from build123d import *

# Parameters (mm, degrees)
BOSS_EXTRUDE1_DEPTH           = 5
SHELL1_T                      = -1
BOSS_EXTRUDE2_DEPTH           = 3.5
CBORE_FOR_M2_SHCS1_AT_2_COUNT = 2
CBORE_FOR_M2_SHCS1_AT_2_PITCH = 23.999204153
FILLET1_R                     = 0.5
SKETCH5_R                     = 5.5
CUT_EXTRUDE1_DEPTH            = 10


with BuildPart() as part:
    # Sketch1 → Boss-Extrude1 (new body)
    with BuildSketch(Plane.XY):
        with BuildLine():
            ThreePointArc((-3.835922715, 7.919955614), (-5.100340344, 7.171229209), (-6.222539674, 6.222539674))
            Line((-6.222539674, 6.222539674), (6.222539674, -6.222539674))
            ThreePointArc((6.222539674, -6.222539674), (7.171229209, -5.100340344), (7.919955614, -3.835922715))
            ThreePointArc((7.919955614, -3.835922715), (8.577167639, -1.967789445), (8.8, 0))
            ThreePointArc((8.8, 0), (4.67353614, 7.456410661), (-3.835922715, 7.919955614))
        make_face()
        with BuildLine():
            Line((6.222539674, -6.222539674), (-6.222539674, 6.222539674))
            ThreePointArc((-6.222539674, 6.222539674), (-7.171229209, 5.100340344), (-7.919955614, 3.835922715))
            ThreePointArc((-7.919955614, 3.835922715), (-6.222539674, -6.222539674), (3.835922715, -7.919955614))
            ThreePointArc((3.835922715, -7.919955614), (5.100340344, -7.171229209), (6.222539674, -6.222539674))
        make_face()
    extrude(amount=BOSS_EXTRUDE1_DEPTH)

    # Shell1
    shell1_openings = [part.faces().sort_by_distance(p)[0] for p in [
        (0, 0, 0),
    ]]
    offset(amount=SHELL1_T, openings=shell1_openings, kind=Kind.INTERSECTION)

    # Sketch1_4 → Boss-Extrude2 (add)
    with BuildSketch(Plane.XY):
        with BuildLine():
            ThreePointArc((-7.919955614, 3.835922715), (-7.171229209, 5.100340344), (-6.222539674, 6.222539674))
            ThreePointArc((-6.222539674, 6.222539674), (-5.100340344, 7.171229209), (-3.835922715, 7.919955614))
            Line((-3.835922715, 7.919955614), (-8.49355603, 12.577588929))
            Line((-8.49355603, 12.577588929), (-12.577588929, 8.49355603))
            Line((-12.577588929, 8.49355603), (-7.919955614, 3.835922715))
        make_face()
        with BuildLine():
            ThreePointArc((7.919955614, -3.835922715), (7.171229209, -5.100340344), (6.222539674, -6.222539674))
            ThreePointArc((6.222539674, -6.222539674), (5.100340344, -7.171229209), (3.835922715, -7.919955614))
            Line((3.835922715, -7.919955614), (8.49355603, -12.577588929))
            Line((8.49355603, -12.577588929), (12.577588929, -8.49355603))
            Line((12.577588929, -8.49355603), (7.919955614, -3.835922715))
        make_face()
    extrude(amount=BOSS_EXTRUDE2_DEPTH)

    # Sketch4 → CBORE for M2 SHCS1 (revolve, cut)
    with BuildSketch(Plane(origin=(-8.485, 8.485, 3.5), x_dir=(0, -1, 0), z_dir=(1, 0, 0))):
        Polygon((0, 0), (0, 3.5), (1.2, 3.5), (1.2, 2), (2.2, 2), (2.2, 0.025), (2.225, 0), align=None)
    cbore_for_m2_shcs1 = revolve(axis=Axis((-8.485, 8.485, 9.85), (0, 0, -1)), mode=Mode.SUBTRACT)

    # CBORE for M2 SHCS1 at 2: CBORE for M2 SHCS1 ×2
    with Locations(*[Vector(0.7071067811865476, -0.7071067811865476, 0) * (i * CBORE_FOR_M2_SHCS1_AT_2_PITCH) for i in range(1, CBORE_FOR_M2_SHCS1_AT_2_COUNT)]):
        add(cbore_for_m2_shcs1, mode=Mode.SUBTRACT)

    # Fillet1
    fillet1_edges = [part.edges().sort_by_distance(p)[0] for p in [
        (6.164739372, -10.248772271, 3.5),
        (8.49355603, -12.577588929, 1.75),
        (12.577588929, -8.49355603, 1.75),
        (10.535572479, -10.535572479, 3.5),
        (10.248772271, -6.164739372, 3.5),
        (-12.577588929, 8.49355603, 1.75),
        (-6.164739372, 10.248772271, 3.5),
        (-8.49355603, 12.577588929, 1.75),
        (-10.248772271, 6.164739372, 3.5),
        (-10.535572479, 10.535572479, 3.5),
        (6.222539674, -6.222539674, 5),
    ]]
    fillet(fillet1_edges, radius=FILLET1_R)

    # Sketch5 → Cut-Extrude1 (cut)
    with BuildSketch(Plane.XY.offset(5)):
        Circle(SKETCH5_R)
    extrude(amount=-CUT_EXTRUDE1_DEPTH, mode=Mode.SUBTRACT)


solid = part.part
For this review, take the finished solid that the model builds, in its own axes (mm). A direction names the side the tool comes from. Round coordinates to 2 decimals unless told otherwise and drop trailing zeros. Use one line per item in the form item = value.
1) Clearance check with flat-ended pins moving along their axes: P1, Ø1.5, axis at y = -8, z = 1, coming from the -X side; P2, Ø2, axis at x = -7.5, y = 7.5, coming from the +Z side; P3, Ø1, axis at x = -2, y = 10, coming from the +Z side; P4, Ø5, axis at x = 1, y = -4.5, coming from the -Z side. State where each tip first meets the part, or that it passes through.
Solutions:
P1 = -4.99
P2 = 3.5
P3 = through
P4 = 4
2) Tool access review of faces 1 (the face through (9.94, -6.06, 3.35)), 2 (the face through (-6.12, 10, 3.35)), 3 (the face through (5.958, -10.042, 1.479)): name each direction out of +Z, -Z, +X, -X, +Y, -Y from which nothing blocks a thin tool from reaching the whole face with its end or side.
Solutions:
face_1 = +Z, +X
face_2 = +Z, +Y
face_3 = +Z, -Z, -Y
3) Wall thickness on probe 1 along Y at (x, z) = (0, 4.4); probe 2 along X at (y, z) = (-4, 1.4); probe 3 along Z at (x, y) = (-1.25, 7.25): over which ranges is each line inside the solid? List them lowest first.
Solutions:
probe_1 = -8.8 to -5.5, 5.5 to 8.8
probe_2 = -7.84 to -6.7, 6.7 to 8.08
probe_3 = 4 to 5
